Could you check a few things on this drawing? It's one solid part, dimensions in mm from its lowest x, y, z. A direction names the side the tool comes from. Give positions to 0.01 mm unless a question says otherwise; leave off trailing zeros. Loops run counter-clockwise (first coordinate to the right, second up) from the corner with the lowest first, then second, coordinate; pieces in that order, holes last. Notation, with made-up numbers: M 82.25,74 L 112.25,74 A10 ccw 112.25,91 Z; hole C 54,76.25 d3. An arc over 180 degrees is marked long. Answer in a Markdown table with one row per item. Add a question column.
1. I'm going to push flat-ended pins straight in: pin 1 Ø1.5 at (y, z) = (6, 26.5) entering from -X; pin 2 Ø8.5 at (y, z) = (18, 9) entering from +X; pin 3 Ø2 at (x, y) = (5.5, 43) entering from +Z. Where does each tip first touch, or does it pass through?
2. Thinking about a two-plate mould opening in Y: for the marked faces 1, 2, 3 and 4, which applies, released by +Y, released by -Y, zero draft, split by the parting line, or undercut?
3. If we section it at C-C on y = 17.5: List the corners of the cut face in (x, z) for me.
4. I need wall thicknesses on line 1 along Y through (x, z) = (22.5, 17); line 2 along X through (y, z) = (37.5, 19); line 3 along Y through (x, z) = (9.5, 21.5) (1 decimal). Which ranges of each line are inside material? Lowest first, please. Write a range as from..to.
5. If we section it at D-D on z = 19.5: List the corners of the cut face in (x, y) for me.
6. If we section it at B-B on z = 5: List the corners of the cut face in (x, y) for me.
7. If we section it at A-A on x = 22: List the corners of the cut face in (y, z) for me.
8. Which directions (+Z, -Z, +X, -X, +Y, -Y) give clear straight access to the entire face, cutting with the end or side of a thin tool? Please do the marked faces 5 and 6.
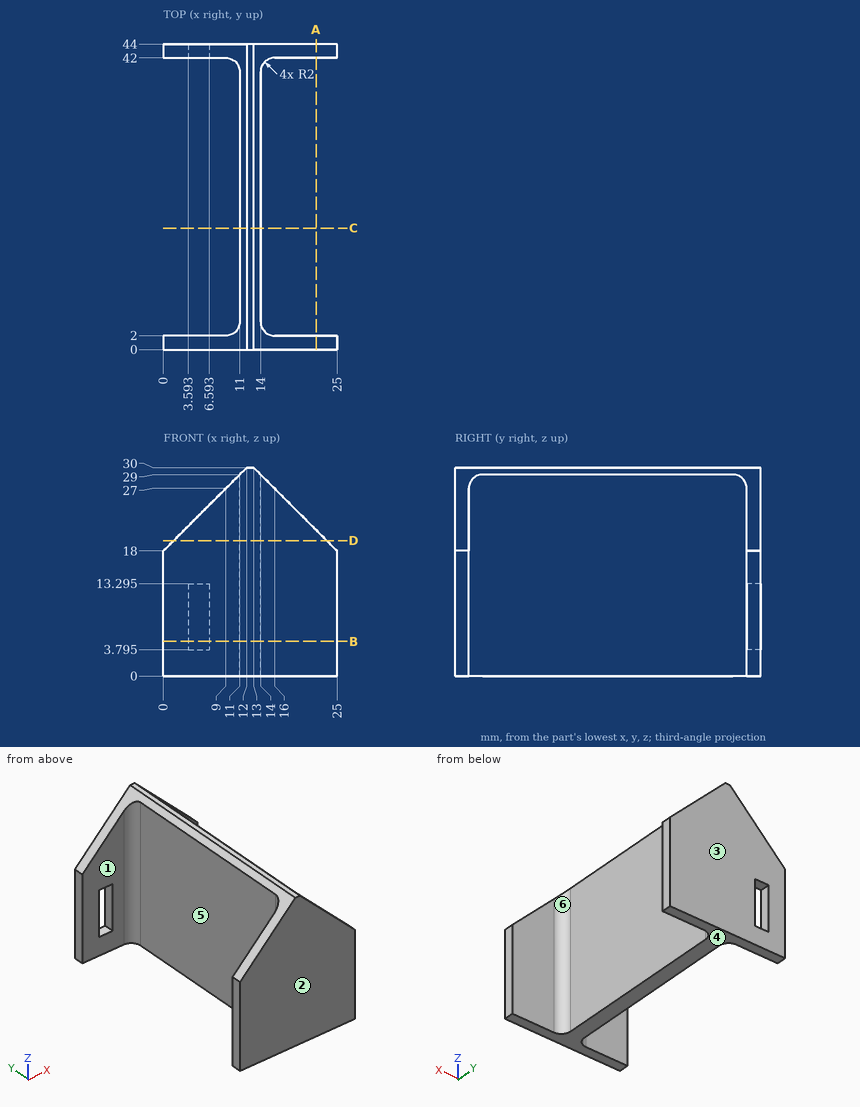
Results:
| question | item | result |
|---|---|---|
| 1 | pin 1 | x = 11 |
| 1 | pin 2 | x = 14 |
| 1 | pin 3 | z = 24.5 |
| 2 | face 1 | undercut |
| 2 | face 2 | released by -Y |
| 2 | face 3 | released by +Y |
| 2 | face 4 | zero draft |
| 3 | outline | M 11,0 L 14,0 L 14,29 L 13,30 L 12,30 L 11,29 Z |
| 4 | line 1 | 0..2, 42..44 |
| 4 | line 2 | 11..14 |
| 4 | line 3 | 0..2.1, 41.9..44 |
| 5 | outline | M 1.5,0 L 23.5,0 L 23.5,2 L 16,2 A2 cw 14,4 L 14,40 A2 cw 16,42 L 23.5,42 L 23.5,44 L 1.5,44 L 1.5,42 L 9,42 A2 cw 11,40 L 11,4 A2 cw 9,2 L 1.5,2 Z |
| 6 | outline | M 0,0 L 25,0 L 25,2 L 16,2 A2 cw 14,4 L 14,40 A2 cw 16,42 L 25,42 L 25,44 L 6.59,44 L 6.59,42 L 9,42 A2 cw 11,40 L 11,4 A2 cw 9,2 L 0,2 Z; M 0,42 L 3.59,42 L 3.59,44 L 0,44 Z |
| 7 | outline | M 0,0 L 2,0 L 2,21 L 0,21 Z; M 42,0 L 44,0 L 44,21 L 42,21 Z |
| 8 | face 5 | +Z, -Z, -X |
| 8 | face 6 | +Z, -Z, +X |
